Input: part model. Units: mm. Frame: model coordinates. Face numbers are marked on the shaded views. A direction names the side the tool comes from. Coordinates: 2 decimals unless noted, no trailing zeros. Write each loop counter-clockwise with the first axis right and the second up, starting at its lowest first coordinate (ties: lowest second). Pieces come first, ordered by that corner, then holes. Notation, with made-up numbers: (25, 2) -> (38, 2) arc R21 cw to (38, 16) -> close; hole circle Ø8 at (48, 87.5). An arc over 180 degrees is marked (long way). Use one line per item in the form item = value. Start each with the question number.
(1) Ray query, line 1 along X through (y, z) = (-3, -8.5); line 2 along X through (y, z) = (1, -9.5); line 3 along Z through (x, y) = (10.5, -1). Return the intervals inside material, ascending.
(2) Cut plane D-D on x = 14.5. Return the cut outline in (y, z), plus the area to 3 significant figures.
(3) Cut plane C-C on x = -3.5. Return the cut outline in (y, z), plus the area to 3 significant figures.
(4) Pull-direction query (X, two-part tool) for the marked faces 1, 2 and 3; classes: released by +X, released by -X, zero draft, split by the parting line, or undercut.
(5) Set-up query: the marked faces 4 and 5. Return all of +Z, -Z, +X, -X, +Y, -Y with unobstructed straight access to the full face (end or side cutting, diameter ignored); none if empty.
(6) Cut plane A-A on z = -5.25. Return the cut outline in (x, y), plus the area to 3 significant figures.
(7) First-contact query: pin 1 (5.5 mm diameter, centred on x = 12, y = -3.5, fed in from -Z); pin 2 (5 mm diameter, centred on x = 10, z = -4, fed in from +Y); pin 3 (1.5 mm diameter, centred on y = -2.5, z = -9.5, fed in from -X); pin 4 (6 mm diameter, centred on x = 9.5, y = -1, fed in from -Z). Flat tips, straight axial feed; report the tip coordinate or a pass-through.
(8) Cut plane B-B on y = 0. Return the cut outline in (x, z), plus the area to 3 significant figures.
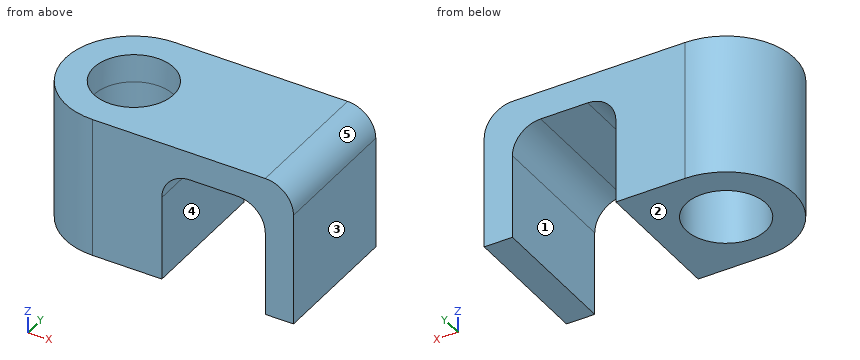
```python
from build123d import *

# Parameters (mm, degrees)
F0_R        = 4.25
F0_W        = 11
F0_H        = 14.5
F0_W_2      = 3
F1_DEPTH    = 3
F2_DEPTH    = 12
F3_T1_DEPTH = 14.5
F3_T3_DEPTH = 29.5
F5_R        = 4.25
F6_DEPTH    = 22
F7_DEPTH    = 3
F8_T1_DEPTH = 28


# Not quite as in the source:
# - a fillet or chamfer that OpenCascade refuses, or shapes differently, is made with other operations: its cross-section is extruded or revolved along the edge and cut away or added


with BuildPart() as f1:
    # F0 (on Top) → F1 (new body)
    with BuildSketch(Plane.XY):
        with BuildLine():
            ThreePointArc((0, -7.25), (5.1265241636, -5.1265241636), (7.25, 0))
            ThreePointArc((7.25, 0), (5.1265241636, 5.1265241636), (0, 7.25))
            ThreePointArc((0, 7.25), (-7.25, 0), (0, -7.25))
        make_face()
        Circle(F0_R, mode=Mode.SUBTRACT)
        with BuildLine():
            Line((7.25, -7.25), (7.25, 0))
            ThreePointArc((7.25, 0), (5.1265241636, -5.1265241636), (0, -7.25))
            Line((0, -7.25), (7.25, -7.25))
        make_face()
        with BuildLine():
            ThreePointArc((0, 7.25), (5.1265241636, 5.1265241636), (7.25, 0))
            Line((7.25, 0), (7.25, 7.25))
            Line((7.25, 7.25), (0, 7.25))
        make_face()
        Polygon((7.25, 7.25), (7.25, 0), (7.25, -7.25), (7.35, -7.25), (7.35, 7.25), align=None)
        with Locations((12.85, 0)):
            Rectangle(F0_W, F0_H)
        with Locations((19.85, 0)):
            Rectangle(F0_W_2, F0_H)
    extrude(amount=F1_DEPTH)

    # F0 (on Top) → F2 (join)
    with BuildSketch(Plane.XY):
        with BuildLine():
            ThreePointArc((0, -7.25), (5.1265241636, -5.1265241636), (7.25, 0))
            ThreePointArc((7.25, 0), (5.1265241636, 5.1265241636), (0, 7.25))
            ThreePointArc((0, 7.25), (-7.25, 0), (0, -7.25))
        make_face()
        Circle(F0_R, mode=Mode.SUBTRACT)
        with BuildLine():
            ThreePointArc((0, 7.25), (5.1265241636, 5.1265241636), (7.25, 0))
            Line((7.25, 0), (7.25, 7.25))
            Line((7.25, 7.25), (0, 7.25))
        make_face()
        Polygon((7.25, 7.25), (7.25, 0), (7.25, -7.25), (7.35, -7.25), (7.35, 7.25), align=None)
        with Locations((19.85, 0)):
            Rectangle(F0_W_2, F0_H)
        with BuildLine():
            Line((7.25, -7.25), (7.25, 0))
            ThreePointArc((7.25, 0), (5.1265241636, -5.1265241636), (0, -7.25))
            Line((0, -7.25), (7.25, -7.25))
        make_face()
    extrude(amount=-F2_DEPTH)

    # F3: fillet of radius 3 on 3 edges, made by hand

    # F3_s2 → F3_t1 (join)
    with BuildSketch(Plane.XZ.offset(-7.25)):
        with BuildLine():
            ThreePointArc((7.35, -3), (8.2286796564, -0.8786796564), (10.35, 0))
            Line((10.35, 0), (7.35, 0))
            Line((7.35, 0), (7.35, -3))
        make_face()
        with BuildLine():
            ThreePointArc((15.35, 0), (17.4713203436, -0.8786796564), (18.35, -3))
            Line((18.35, -3), (18.35, 0))
            Line((18.35, 0), (15.35, 0))
        make_face()
    extrude(amount=F3_T1_DEPTH)

    # F3_s4 → F3_t3 (cut)
    with BuildSketch(Plane.XZ.offset(-14.75)):
        with BuildLine():
            ThreePointArc((18.35, 3), (20.4713203436, 2.1213203436), (21.35, 0))
            Line((21.35, 0), (21.35, 3))
            Line((21.35, 3), (18.35, 3))
        make_face()
    extrude(amount=F3_T3_DEPTH, mode=Mode.SUBTRACT)


with BuildPart() as f6:
    # F5 (on offset) → F6 (new body)
    with BuildSketch(Plane(origin=(0, 0, -37), x_dir=(1, 0, 0), z_dir=(0, 0, -1))):
        with BuildLine():
            Line((7.35, 7.25), (0, 7.25))
            ThreePointArc((0, 7.25), (-7.25, 0), (0, -7.25))
            Line((0, -7.25), (7.35, -7.25))
            Line((7.35, -7.25), (7.35, 7.25))
        make_face()
        Circle(F5_R, mode=Mode.SUBTRACT)
    extrude(amount=-F6_DEPTH)

    # F5 (on offset) → F7 (join)
    with BuildSketch(Plane(origin=(0, 0, -37), x_dir=(1, 0, 0), z_dir=(0, 0, -1))):
        with BuildLine():
            Line((7.35, 7.25), (0, 7.25))
            ThreePointArc((0, 7.25), (-7.25, 0), (0, -7.25))
            Line((0, -7.25), (7.35, -7.25))
            Line((7.35, -7.25), (7.35, 7.25))
        make_face()
        Circle(F5_R, mode=Mode.SUBTRACT)
        with BuildLine():
            ThreePointArc((0, -7.25), (-7.25, 0), (0, 7.25))
            Line((0, 7.25), (-37.25, 7.25))
            Line((-37.25, 7.25), (-37.25, 4))
            Line((-37.25, 4), (-22.25, 4))
            ThreePointArc((-22.25, 4), (-18.25, 0), (-22.25, -4))
            Line((-22.25, -4), (-37.25, -4))
            Line((-37.25, -4), (-37.25, -7.25))
            Line((-37.25, -7.25), (0, -7.25))
        make_face()
    extrude(amount=F7_DEPTH)

    # F8: fillet of radius 5 on 2 edges, made by hand

    # F8_s2 → F8_t1 (cut)
    with BuildSketch(Plane.XY.offset(-52.5)):
        with BuildLine():
            ThreePointArc((-32.25, -7.25), (-35.7855339059, -5.7855339059), (-37.25, -2.25))
            Line((-37.25, -2.25), (-37.25, -7.25))
            Line((-37.25, -7.25), (-32.25, -7.25))
        make_face()
        with BuildLine():
            ThreePointArc((-32.25, 7.25), (-35.7855339059, 5.7855339059), (-37.25, 2.25))
            Line((-37.25, 2.25), (-37.25, 7.25))
            Line((-37.25, 7.25), (-32.25, 7.25))
        make_face()
    extrude(amount=F8_T1_DEPTH, mode=Mode.SUBTRACT)


solid = f1.part
```
Values:
q1.line_1 = -6.6 to -3.01, 3.01 to 7.35, 18.35 to 21.35
q1.line_2 = -7.18 to -4.13, 4.13 to 7.35, 18.35 to 21.35
q1.line_3 = 0 to 3
q2.outline = (-7.25, 0) -> (7.25, 0) -> (7.25, 3) -> (-7.25, 3) -> close
q2.area = 43.5 mm2
q3.outline = (-6.35, -12) -> (-2.41, -12) -> (-2.41, 3) -> (-6.35, 3) -> close; (2.41, -12) -> (6.35, -12) -> (6.35, 3) -> (2.41, 3) -> close
q3.area = 118 mm2
q4.face_1 = undercut
q4.face_2 = zero draft
q4.face_3 = released by +X
q5.face_4 = -Z, +Y, -Y
q5.face_5 = +Z, +X, +Y, -Y
q6.outline = (0, -7.25) -> (7.35, -7.25) -> (7.35, 7.25) -> (0, 7.25) arc R7.25 ccw to start; (18.35, -7.25) -> (21.35, -7.25) -> (21.35, 7.25) -> (18.35, 7.25) -> close; hole circle Ø8.5 at (0, 0)
q6.area = 176 mm2
q7.pin_1 = -0.21
q7.pin_2 = through
q7.pin_3 = -7.04
q7.pin_4 = -12
q8.outline = (-7.25, -12) -> (-4.25, -12) -> (-4.25, 3) -> (-7.25, 3) -> close; (4.25, -12) -> (7.35, -12) -> (7.35, -3) arc R3 cw to (10.35, 0) -> (15.35, 0) arc R3 cw to (18.35, -3) -> (18.35, -12) -> (21.35, -12) -> (21.35, 0) arc R3 ccw to (18.35, 3) -> (4.25, 3) -> close
q8.area = 171 mm2
